The listing builds one solid part. Answer for the finished solid, in the listing's coordinates (mm). A direction names the side the tool comes from. Give positions to 0.01 mm unless a question says otherwise; leave off trailing zeros. Write each loop counter-clockwise with the first axis right and the second up, starting at its lowest first coordinate (ties: lowest second). Pieces come first, ordered by that corner, then holes. Notation, with made-up numbers: M -34.75,-9.5 L -7.75,-9.5 A13 ccw -7.75,10.5 Z; hole C -40,3 d9. An arc over 180 degrees is marked long. Answer as a JSON object with one key per item and string values.
```python
from build123d import *

# Parameters (mm, degrees)
ESQUISSE1_R             = 2
BOSS_EXTRU_1_DEPTH      = 24
ESQUISSE2_R             = 2.5
BOSS_EXTRU_2_DEPTH      = 36.5
CHANFREIN1_SIZE         = 0.5
TROU_TARAUD_M1_61_D     = 1.25
TROU_TARAUD_M1_61_DEPTH = 4.95
TROU_TARAUD_M1_61_TIP   = 0.375537887
ENL_V_START             = -15
ENL_V_MAT_EXTRU_1_DEPTH = 15
CHANFREIN2_SIZE         = 0.25


with BuildPart() as part:
    # Esquisse1 → Boss.-Extru.1 (new body)
    with BuildSketch(Plane(origin=(0, 0, 0), x_dir=(1, 0, 0), z_dir=(0, 1, 0))):
        with Locations(Location((0, 0, 0), (0, 0, 270))):
            Circle(ESQUISSE1_R)
    extrude(amount=BOSS_EXTRU_1_DEPTH)

    # Esquisse2 → Boss.-Extru.2 (add)
    with BuildSketch(Plane.XZ):
        with Locations(Location((0, 0, 0), (0, 0, 270))):
            Circle(ESQUISSE2_R)
    extrude(amount=BOSS_EXTRU_2_DEPTH)

    # Chanfrein1
    chanfrein1_edges = [part.edges().sort_by_distance(p)[0] for p in [
        (0, 24, -2),
    ]]
    chamfer(chanfrein1_edges, length=CHANFREIN1_SIZE)

    # Trou taraudé M1.61
    with Locations(Plane(origin=(0, 24, 0), x_dir=(1, 0, 0), z_dir=(0, 1, 0))):
        with Locations((0, 0)):
            Hole(TROU_TARAUD_M1_61_D / 2, depth=TROU_TARAUD_M1_61_DEPTH)
            with Locations((0, 0, -(TROU_TARAUD_M1_61_DEPTH + TROU_TARAUD_M1_61_TIP / 2))):  # 118° drill point
                Cone(0, TROU_TARAUD_M1_61_D / 2, TROU_TARAUD_M1_61_TIP, mode=Mode.SUBTRACT)

    # Esquisse5 → Enlèv. mat.-Extru.1 (cut)
    with BuildSketch(Plane(origin=(0, 24, 0), x_dir=(1, 0, 0), z_dir=(0, 1, 0)).offset(ENL_V_START)):
        with BuildLine():
            Line((-1.322875656, 1.5), (1.322875656, 1.5))
            ThreePointArc((1.322875656, 1.5), (0, 2), (-1.322875656, 1.5))
        make_face()
    extrude(amount=ENL_V_MAT_EXTRU_1_DEPTH, mode=Mode.SUBTRACT)

    # Chanfrein2
    chanfrein2_edges = [part.edges().sort_by_distance(p)[0] for p in [
        (0, 0, 2.5),
        (0, -36.5, 2.5),
    ]]
    chamfer(chanfrein2_edges, length=CHANFREIN2_SIZE)


solid = part.part
```
1. The mould has two halves that part along X. Classify faces 4 (the conical face through (-0.02, 18.74, 0.11)), 5 (the cylindrical face through (-2.44, -18, 0.54)), 6 (the flat face through (0, 24, 1)): released by +X, released by -X, zero draft, split by the parting line, or undercut.
Verdict:
{"face 4": "undercut", "face 5": "split by the parting line", "face 6": "zero draft"}
2. A cutting plane is placed at A-A, the plane y = -4. Give the vertices of the cut face in (x, z), plus the area to 3 significant figures.
Verdict:
{"outline": "C 0,0 d5", "area": "19.6 mm2"}
3. Consider line 1 along Z through (x, y) = (0, 22.6) (3 decimals); line 2 along Z through (x, y) = (2, -20.5); line 3 along Y through (x, z) = (2.05, -0.7). Determine where each line is inside the solid, lowest interval first.
Verdict:
{"line 1": "z = -1.5 to -0.625, 0.625 to 2", "line 2": "z = -1.5 to 1.5", "line 3": "y = -36.5 to 0"}
4. For faces 1 (the flat face through (0, 16, -1.5)), 2 (the flat face through (0, -36.5, 0)), 3 (the cylindrical face through (0.14, 21.49, 0.61)), determine the directions among +Z, -Z, +X, -X, +Y, -Y from which every point of the face is accessible in a straight line to the end or side of a thin tool.
Verdict:
{"face 1": "-Z, +X, -X, +Y", "face 2": "+Z, -Z, +X, -X, -Y", "face 3": "+Y"}
5. A cutting plane is placed at B-B, the plane y = 6. Give the vertices of the cut face in (x, z), plus the area to 3 significant figures.
Verdict:
{"outline": "C 0,0 d4", "area": "12.6 mm2"}
6. Flat-ended cylindrical pins translate along their axes: pin 1 (1.5 mm diameter, centred on x = 2, y = -29.5, fed in from -Z); pin 2 (1 mm diameter, centred on y = 7, z = 1.5, fed in from +X); pin 3 (2 mm diameter, centred on x = 0, y = 15, fed in from -Z). Find the tip coordinate at first contact, or state that the pin passes through.
Verdict:
{"pin 1": "stops at z = -2.17", "pin 2": "stops at x = 1.73", "pin 3": "stops at z = -1.5"}
